The listing builds one solid part. Answer for the finished solid, in the listing's coordinates (mm). A direction names the side the tool comes from. Round coordinates to 2 decimals unless told otherwise and drop trailing zeros. Loops run counter-clockwise (first coordinate to the right, second up) from the corner with the lowest first, then second, coordinate; pieces in that order, holes last. Notation, with made-up numbers: (-25.75, -21) -> (-8.75, -21) arc R8 ccw to (-8.75, -11) -> close; hole circle Ø11 at (80, 61.25). An arc over 180 degrees is marked (long way). One line per question, with ' | ' between items.
Autodesk Inventor part; units mm, degrees
ref_plane "Work Plane1" through (0, 25, 8.75) normal (0, 0, 1) x (1, 0, 0)
ref_plane "YZ Plane" through (0, 0, 0) normal (1, 0, 0) x (0, 1, 0)
ref_plane "XZ Plane" through (0, 0, 0) normal (0, 1, 0) x (-1, 0, 0)
sketch "Sketch1" plane through (0, 0, 0) normal (1, 0, 0) x (0, 1, 0)
  line L0 (80, 41.5) -> (25, 41.5)
  line L1 (25, 41.5) -> (25, -10)
  line L2 (25, -10) -> (80, -10)
  line L3 (80, -10) -> (80, 41.5)
  line L4 (25, 0) -> (0, 0)
  line L5 (0, 0) -> (0, -10)
  line L6 (0, -10) -> (25, -10)
  line L7 (25, -10) -> (25, 0)
  line L8 (40, 10) -> (80, 10)
  line L9 (80, 10) -> (80, -10)
  line L10 (80, -10) -> (40, -10)
  line L11 (40, -10) -> (40, 10)
  point P0 (25, -10)
  dimension "d0" = 55
  dimension "d1" = 10
  dimension "d3" = 51.5
  dimension "d135" = 25
  dimension "d144" = 20
  dimension "d145" = 40
extrude "Extrusion1" add sketch "Sketch1" along normal blind 50 contours L3 L8 L11 L2 L1 L0 | L1 L6 L5 L4
ref_plane "Work Plane1" through (0, 25, 8.75) normal (0, 0, 1) x (1, 0, 0)
sketch "Sketch23" plane through (0, 25, 41.5) normal (0, 0, 1) x (1, 0, 0)
  line L0 (38.5, 9.5) -> (11.5, 9.5)
  line L1 (0, 0) -> (50, 0)
  line L2 (38.5, 9.5) -> (38.5, 5.5)
  line L3 (38.5, 5.5) -> (36, 5.5)
  line L4 (36, 5.5) -> (36, 0)
  line L5 (0, 0) -> (50, 0)
  line L6 (11.5, 9.5) -> (11.5, 5.5)
  line L7 (11.5, 5.5) -> (14, 5.5)
  line L8 (14, 5.5) -> (14, 0)
  point P0 (0, -25)
  point P1 (25, 9.5)
  point P2 (25, 0)
  point P3 (14, 0)
  point P4 (36, 0)
  dimension "d149" = 9.5
  dimension "d150" = 4
  dimension "d151" = 2.5
  dimension "d152" = 27
extrude "Extrusion16" cut sketch "Sketch23" against normal up to surface (41.5 mm away)
sketch "Sketch24" plane through (50, 0, 0) normal (1, 0, 0) x (0, 0, -1)
  line L0 (-20, 45) -> (-41.5, 45)
  line L1 (-41.5, 45) -> (-41.5, 80)
  line L2 (-41.5, 80) -> (-20, 80)
  line L3 (-20, 80) -> (-20, 45)
  line L4 (-10, 40) -> (-10, 80)
  line L5 (10, 40) -> (-10, 40)
  line L6 (-41.5, 80) -> (-41.5, 25)
  line L7 (-10, 80) -> (-41.5, 80)
  point P0 (0, 0)
  dimension "d155" = 10
  dimension "d156" = 5
extrude "Extrusion17" cut sketch "Sketch24" against normal through all
sketch "Sketch25" plane through (0, 0, 0) normal (0, 0, 1) x (1, 0, 0)
  circle A0 centre (7.5, 15.5) radius 2.5
  circle A1 centre (42.5, 15.5) radius 2.5
  line L0 (0, 0) -> (50, 0)
  line L1 (50, 25) -> (50, 0)
  dimension "d162" = 5
  dimension "d163" = 15.5
  dimension "d164" = 7.5
  dimension "d165" = 35
hole "Hole5" at (7.5, 15.5, 0) at (42.5, 15.5, 0) direction (0, 0, -1) diameter 5 end through all counterbore diameter 9 counterbore depth 2
move faces "Move6" translate (0, -5, 0) faces at (33.3333, 45, 34.3333)
sketch "Sketch26" plane through (0, 80, 20) normal (0, 0, 1) x (1, 0, 0)
  line L0 (38, -31.5) -> (38, -28.5) construction
  line L1 (41, -31.5) -> (41, -28.5)
  line L2 (35, -28.5) -> (35, -31.5)
  arc A0 (35, -31.5) -> (41, -31.5) centre (38, -31.5) ccw
  arc A1 (41, -28.5) -> (35, -28.5) centre (38, -28.5) ccw
  line L3 (12, -31.5) -> (12, -28.5) construction
  line L4 (15, -31.5) -> (15, -28.5)
  line L5 (9, -28.5) -> (9, -31.5)
  arc A2 (9, -31.5) -> (15, -31.5) centre (12, -31.5) ccw
  arc A3 (15, -28.5) -> (9, -28.5) centre (12, -28.5) ccw
  line L6 (38, -11.5) -> (38, -8.5) construction
  line L7 (41, -11.5) -> (41, -8.5)
  line L8 (35, -8.5) -> (35, -11.5)
  arc A4 (35, -11.5) -> (41, -11.5) centre (38, -11.5) ccw
  arc A5 (41, -8.5) -> (35, -8.5) centre (38, -8.5) ccw
  line L9 (12, -11.5) -> (12, -8.5) construction
  line L10 (15, -11.5) -> (15, -8.5)
  line L11 (9, -8.5) -> (9, -11.5)
  arc A6 (9, -11.5) -> (15, -11.5) centre (12, -11.5) ccw
  arc A7 (15, -8.5) -> (9, -8.5) centre (12, -8.5) ccw
  line L12 (50, 0) -> (50, -35)
  line L13 (0, -35) -> (0, 0)
  line L14 (0, 0) -> (50, 0)
  line L15 (50, -40) -> (0, -40)
  point P0 (0, -80)
  point P1 (38, -30)
  point P2 (12, -30)
  point P3 (38, -10)
  point P4 (12, -10)
  dimension "d173" = 3
  dimension "d174" = 6
  dimension "d176" = 12
  dimension "d177" = 12
  dimension "d178" = 10
  dimension "d185" = 10
extrude "Extrusion18" cut sketch "Sketch26" against normal through all
equation "\"d177\" = d176"
properties part number "10-03-029"
Q1. Given pin 1 Ø1.5 at (x, z) = (16.5, 11.5) entering from -Y; pin 2 Ø21.5 at (x, z) = (25.5, 29.5) entering from -Y; pin 3 Ø5 at (x, y) = (23.5, 68) entering from -Z, each flat-ended and moving along its own axis, determine where each tip first touches the part or whether it passes through.
Numbers:
pin 1: y = 34.5 | pin 2: y = 25 | pin 3: z = 10
Q2. Find the intervals of material crossed by line 1 (X direction, y = 15.5, z = -0.5); line 2 (X direction, y = 15.5, z = -5.25); line 3 (Y direction, x = 37, z = 31), in increasing order. Write a range as from..to.
Numbers:
line 1: 0..3, 12..38, 47..50 | line 2: 0..5, 10..40, 45..50 | line 3: 25..30.5, 34.5..40
Q3. A cutting plane is placed at B-B on x = 42.5. Give the vertices of the cut face in (y, z).
Numbers:
outline: (0, -10) -> (13, -10) -> (13, -2) -> (11, -2) -> (11, 0) -> (0, 0) -> close; (18, -10) -> (40, -10) -> (40, 10) -> (80, 10) -> (80, 20) -> (40, 20) -> (40, 41.5) -> (25, 41.5) -> (25, 0) -> (20, 0) -> (20, -2) -> (18, -2) -> close
Q4. A cutting plane is placed at C-C on z = -4.5. Give the vertices of the cut face in (x, y), plus the area to 3 significant figures.
Numbers:
outline: (0, 0) -> (50, 0) -> (50, 40) -> (0, 40) -> close; hole circle Ø5 at (7.5, 15.5); hole circle Ø5 at (42.5, 15.5) | area: 1,960 mm^2
Q5. A cutting plane is placed at A-A on y = 15.5. Give the vertices of the cut face in (x, z).
Numbers:
outline: (0, -10) -> (5, -10) -> (5, -2) -> (3, -2) -> (3, 0) -> (0, 0) -> close; (10, -10) -> (40, -10) -> (40, -2) -> (38, -2) -> (38, 0) -> (12, 0) -> (12, -2) -> (10, -2) -> close; (45, -10) -> (50, -10) -> (50, 0) -> (47, 0) -> (47, -2) -> (45, -2) -> close
Q6. For a pull along X with two mould halves and no side action, classify faces 5 (the face through (35, 70, 15)), 6 (the face through (41, 70, 15)), 7 (the face through (25, 80, 15)), 8 (the face through (0, 39, 10)) as pulls with the +X half, pulls with the -X half, needs draft (parallel to the pull), parting line crosses it, or undercut.
Numbers:
face 5: undercut | face 6: undercut | face 7: needs draft | face 8: pulls with the -X half
Q7. For faces 1 (the face through (14, 28, 21)), 2 (the face through (37.9, 65.5, 15.1)), 3 (the face through (25, 60, 20)), 4 (the face through (38.5, 33, 21)), determine the directions among +Z, -Z, +X, -X, +Y, -Y from which every point of the face is accessible in a straight line to the end or side of a thin tool.
Numbers:
face 1: +Z, -Y | face 2: +Z, -Z | face 3: +Z, +X, -X, +Y | face 4: +Z
Q8. A cutting plane is placed at D-D on z = 13. Give the vertices of the cut face in (x, y), plus the area to 3 significant figures.
Numbers:
outline: (0, 25) -> (14, 25) -> (14, 30.5) -> (11.5, 30.5) -> (11.5, 34.5) -> (38.5, 34.5) -> (38.5, 30.5) -> (36, 30.5) -> (36, 25) -> (50, 25) -> (50, 80) -> (0, 80) -> close; hole (9, 48.5) arc R3 ccw to (15, 48.5) -> (15, 51.5) arc R3 ccw to (9, 51.5) -> close; hole (9, 68.5) arc R3 ccw to (15, 68.5) -> (15, 71.5) arc R3 ccw to (9, 71.5) -> close; hole (35, 48.5) arc R3 ccw to (41, 48.5) -> (41, 51.5) arc R3 ccw to (35, 51.5) -> close; hole (35, 68.5) arc R3 ccw to (41, 68.5) -> (41, 71.5) arc R3 ccw to (35, 71.5) -> close | area: 2,340 mm^2
